The figure shows three views and two pictorial views of one solid part (mm, origin at its lowest corner). Answer the questions. Round coordinates to 2 decimals unless told otherwise and drop trailing zeros. Order: outer loops, then holes, each group sorted by start corner. A loop starts at its lowest first (then second) coordinate and runs counter-clockwise, first axis right, second up. Notation, with made-up numbers: (-29, 39) - (-19, 39) arc R23 ccw to (-19, 50) - close; hole circle Ø6 at (25, 75.5). An arc over 180 degrees is marked (long way). One line per item, written item: value. Start each with the question number.
1. Section B-B, the plane x = 12 is taken. Give the vertices of the cut face in (y, z) (1 decimal).
2. Flat-ended cylindrical pins translate along their axes: P1, Ø2.5, axis at x = 8.63, y = 13.75, coming from the +Z side; P2, Ø3, axis at y = 37.5, z = 3.5, coming from the +X side; P3, Ø2, axis at y = 26.5, z = 3.5, coming from the -X side; P4, Ø2, axis at y = 28.5, z = 3.5, coming from the -X side. Find the tip coordinate at first contact, or state that the pin passes through.
3. Section D-D, the plane z = 2.4 is taken. Count the separate pieces of the cut face and the enclosed holes in it, then the cut area to 3 significant figures.
4. Straight lines are drawn through the part: line 1 (Y direction, x = 20.75, z = 3.25); line 2 (X direction, y = 27.5, z = 4.8) (1 decimal); line 3 (Y direction, x = 22, z = 3.3) (1 decimal). For each, find the intervals that lie inside material, in ascending order.
5. Section C-C, the plane y = 24 is taken. Give the vertices of the cut face in (x, z).
6. Section A-A, the plane y = 13.75 is taken. Give the vertices of the cut face in (x, z) (1 decimal).
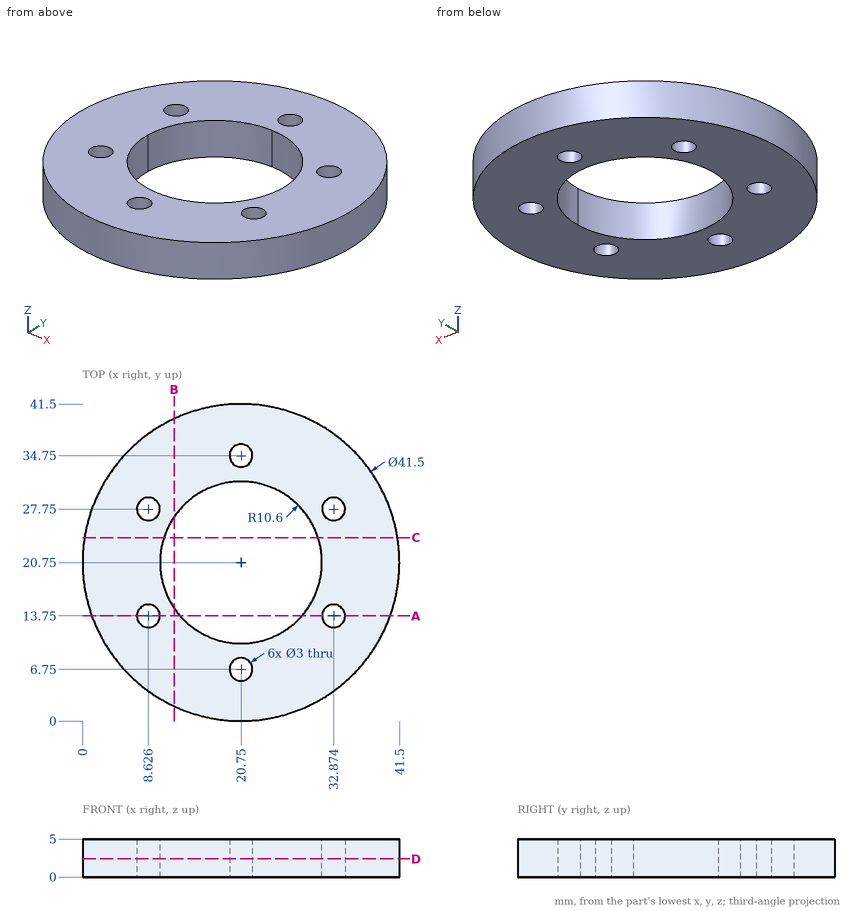
Answer list:
1. outline: (1.9, 0) - (14.8, 0) - (14.8, 5) - (1.9, 5) - close; (26.7, 0) - (39.6, 0) - (39.6, 5) - (26.7, 5) - close
2. P1: passes through
2. P2: stops at x = 34.82
2. P3: stops at x = 0.55
2. P4: stops at x = 1.13
3. separate pieces: 1
3. enclosed holes: 7
3. area: 957 mm²
4. line 1: y = 0 to 5.25, 8.25 to 10.15, 31.35 to 33.25, 36.25 to 41.5
4. line 2: x = 1.1 to 7.1, 10.1 to 12.6, 28.9 to 31.4, 34.4 to 40.4
4. line 3: y = 0 to 5.9, 7.6 to 10.2, 31.3 to 33.9, 35.6 to 41.5
5. outline: (0.26, 0) - (10.66, 0) - (10.66, 5) - (0.26, 5) - close; (30.84, 0) - (41.24, 0) - (41.24, 5) - (30.84, 5) - close
6. outline: (1.2, 0) - (7.1, 0) - (7.1, 5) - (1.2, 5) - close; (10.1, 0) - (12.8, 0) - (12.8, 5) - (10.1, 5) - close; (28.7, 0) - (31.4, 0) - (31.4, 5) - (28.7, 5) - close; (34.4, 0) - (40.3, 0) - (40.3, 5) - (34.4, 5) - close
